Could you check a few things on this model? Use its own coordinates, in mm. A direction names the side the tool comes from. Coordinates: 2 decimals unless noted, no trailing zeros. Loops run counter-clockwise (first coordinate to the right, second up) from the corner with the lowest first, then second, coordinate; pieces in that order, holes last. Notation, with made-up numbers: (42.25, 40.25) - (101.25, 40.25) arc R30 cw to (101.25, 77.25) - close; hole circle Ø6 at (68.5, 56.5). An arc over 180 degrees is marked (long way). Use CSV: the item, a comma, the result in double quotes.
from build123d import *

# Parameters (mm, degrees)
BOSS_EXTRUDE1_DEPTH = 3
BOSS_EXTRUDE2_DEPTH = 13
FILLET1_R           = 10


with BuildPart() as part:
    # Sketch1 → Boss-Extrude1 (new body)
    with BuildSketch(Plane.XY):
        with BuildLine():
            ThreePointArc((44.504151191, -3.633742271), (52.754151191, 4.616257729), (61.004151191, -3.633742271))
            Line((61.004151191, -3.633742271), (71.117527312, -3.633742271))
            Line((71.117527312, -3.633742271), (71.117527312, 12.71809795))
            Line((71.117527312, 12.71809795), (-33.093009972, 12.71809795))
            Line((-33.093009972, 12.71809795), (-33.093009972, -3.633742271))
            Line((-33.093009972, -3.633742271), (-21.941421773, -3.633742271))
            ThreePointArc((-21.941421773, -3.633742271), (-13.691421773, 4.616257729), (-5.441421773, -3.633742271))
            Line((-5.441421773, -3.633742271), (10.76225867, -3.633742271))
            ThreePointArc((10.76225867, -3.633742271), (19.01225867, 4.616257729), (27.26225867, -3.633742271))
            Line((27.26225867, -3.633742271), (44.504151191, -3.633742271))
        make_face()
        with BuildLine():
            Line((71.117527312, -3.633742271), (61.004151191, -3.633742271))
            ThreePointArc((61.004151191, -3.633742271), (52.754151191, -11.883742271), (44.504151191, -3.633742271))
            Line((44.504151191, -3.633742271), (27.26225867, -3.633742271))
            ThreePointArc((27.26225867, -3.633742271), (19.01225867, -11.883742271), (10.76225867, -3.633742271))
            Line((10.76225867, -3.633742271), (-5.441421773, -3.633742271))
            ThreePointArc((-5.441421773, -3.633742271), (-13.691421773, -11.883742271), (-21.941421773, -3.633742271))
            Line((-21.941421773, -3.633742271), (-33.093009972, -3.633742271))
            Line((-33.093009972, -3.633742271), (-33.093009972, -19.985582493))
            Line((-33.093009972, -19.985582493), (71.117527312, -19.985582493))
            Line((71.117527312, -19.985582493), (71.117527312, -3.633742271))
        make_face()
        with BuildLine():
            ThreePointArc((-21.941421773, -3.633742271), (-13.691421773, -11.883742271), (-5.441421773, -3.633742271))
            Line((-5.441421773, -3.633742271), (-21.941421773, -3.633742271))
        make_face()
        with BuildLine():
            Line((-21.941421773, -3.633742271), (-5.441421773, -3.633742271))
            ThreePointArc((-5.441421773, -3.633742271), (-13.691421773, 4.616257729), (-21.941421773, -3.633742271))
        make_face()
        with BuildLine():
            ThreePointArc((10.76225867, -3.633742271), (19.01225867, -11.883742271), (27.26225867, -3.633742271))
            Line((27.26225867, -3.633742271), (10.76225867, -3.633742271))
        make_face()
        with BuildLine():
            Line((10.76225867, -3.633742271), (27.26225867, -3.633742271))
            ThreePointArc((27.26225867, -3.633742271), (19.01225867, 4.616257729), (10.76225867, -3.633742271))
        make_face()
        with BuildLine():
            ThreePointArc((44.504151191, -3.633742271), (52.754151191, -11.883742271), (61.004151191, -3.633742271))
            Line((61.004151191, -3.633742271), (44.504151191, -3.633742271))
        make_face()
        with BuildLine():
            Line((44.504151191, -3.633742271), (61.004151191, -3.633742271))
            ThreePointArc((61.004151191, -3.633742271), (52.754151191, 4.616257729), (44.504151191, -3.633742271))
        make_face()
    extrude(amount=BOSS_EXTRUDE1_DEPTH)

    # Sketch1_3 → Boss-Extrude2 (add)
    with BuildSketch(Plane.XY):
        with BuildLine():
            ThreePointArc((-21.941421773, -3.633742271), (-13.691421773, -11.883742271), (-5.441421773, -3.633742271))
            Line((-5.441421773, -3.633742271), (-21.941421773, -3.633742271))
        make_face()
        with BuildLine():
            Line((-21.941421773, -3.633742271), (-5.441421773, -3.633742271))
            ThreePointArc((-5.441421773, -3.633742271), (-13.691421773, 4.616257729), (-21.941421773, -3.633742271))
        make_face()
        with BuildLine():
            ThreePointArc((10.76225867, -3.633742271), (19.01225867, -11.883742271), (27.26225867, -3.633742271))
            Line((27.26225867, -3.633742271), (10.76225867, -3.633742271))
        make_face()
        with BuildLine():
            Line((10.76225867, -3.633742271), (27.26225867, -3.633742271))
            ThreePointArc((27.26225867, -3.633742271), (19.01225867, 4.616257729), (10.76225867, -3.633742271))
        make_face()
        with BuildLine():
            ThreePointArc((44.504151191, -3.633742271), (52.754151191, -11.883742271), (61.004151191, -3.633742271))
            Line((61.004151191, -3.633742271), (44.504151191, -3.633742271))
        make_face()
        with BuildLine():
            Line((44.504151191, -3.633742271), (61.004151191, -3.633742271))
            ThreePointArc((61.004151191, -3.633742271), (52.754151191, 4.616257729), (44.504151191, -3.633742271))
        make_face()
    extrude(amount=BOSS_EXTRUDE2_DEPTH)

    # Fillet1
    fillet1_edges = [part.edges().sort_by_distance(p)[0] for p in [
        (-33.093009972, -19.985582493, 1.5),
        (-33.093009972, 12.71809795, 1.5),
        (71.117527312, 12.71809795, 1.5),
        (71.117527312, -19.985582493, 1.5),
    ]]
    fillet(fillet1_edges, radius=FILLET1_R)

    # Fillet2: read off the stored shape, not the designer's step
    # Fillet2 outline → Fillet2 (revolve, cut)
    with BuildSketch(Plane(origin=(52.754151191, -3.633742271, 0), x_dir=(1, 0, 0), z_dir=(0, -1, 0))):
        with BuildLine():
            ThreePointArc((5.75, 13), (7.517766953, 12.267766953), (8.25, 10.5))
            Line((8.25, 10.5), (8.25, 13))
            Line((8.25, 13), (5.75, 13))
        make_face()
    revolve(axis=Axis((52.754151191, -3.633742271, 0), (0, 0, 1)), mode=Mode.SUBTRACT)

    # Fillet2 2 outline → Fillet2 2 (revolve, cut)
    with BuildSketch(Plane(origin=(19.01225867, -3.633742271, 0), x_dir=(1, 0, 0), z_dir=(0, -1, 0))):
        with BuildLine():
            ThreePointArc((5.75, 13), (7.517766953, 12.267766953), (8.25, 10.5))
            Line((8.25, 10.5), (8.25, 13))
            Line((8.25, 13), (5.75, 13))
        make_face()
    revolve(axis=Axis((19.01225867, -3.633742271, 0), (0, 0, 1)), mode=Mode.SUBTRACT)

    # Fillet2 3 outline → Fillet2 3 (revolve, cut)
    with BuildSketch(Plane(origin=(-13.691421773, -3.633742271, 0), x_dir=(1, 0, 0), z_dir=(0, -1, 0))):
        with BuildLine():
            ThreePointArc((5.75, 13), (7.517766953, 12.267766953), (8.25, 10.5))
            Line((8.25, 10.5), (8.25, 13))
            Line((8.25, 13), (5.75, 13))
        make_face()
    revolve(axis=Axis((-13.691421773, -3.633742271, 0), (0, 0, 1)), mode=Mode.SUBTRACT)


solid = part.part
(1) Suppose I cut it at B-B (z = 11.75). Write out the boundary of the cut face in (x, y).
Computed:
outline,"circle Ø15.83 at (-13.69, -3.63); circle Ø15.83 at (19.01, -3.63); circle Ø15.83 at (52.75, -3.63)"
(2) Thinking about a two-plate mould opening in X: for faces 3 (the face through (18, -19.986, 1)), 4 (the face through (-9.256, 3.323, 6.698)), 5 (the face through (71.118, -4, 1)), which applies, +X half, -X half, draft (parallel to the pull), parting line (faces both ways), or undercut?
Computed:
face 3,"draft"
face 4,"undercut"
face 5,"+X half"
(3) Please list where these lines run through material, in increasing order: line 1 (X direction, y = -9, z = 8.75); line 2 (X direction, y = -8.5, z = 6.5); line 3 (Z direction, x = 67.5, y = 0.5).
Computed:
line 1,"x = -19.96 to -7.43, 12.75 to 25.28, 46.49 to 59.02"
line 2,"x = -20.35 to -7.03, 12.35 to 25.67, 46.09 to 59.42"
line 3,"z = 0 to 3"
(4) Which directions (+Z, -Z, +X, -X, +Y, -Y) give clear straight access to the entire face, cutting with the end or side of a thin tool? Please do faces 1 (the face through (-30.086, 9.866, 1.521)), 2 (the face through (44.512, -3.271, 6.698)).
Computed:
face 1,"+Z, -Z, -X, +Y"
face 2,"+Z"
(5) Will these pins go through, and if not, where does the flat tip stop? pin 1 (10 mm diameter, centred on x = -4.5, y = -9.5, fed in from +Z); pin 2 (4 mm diameter, centred on x = 28.5, y = -13, fed in from +Z).
Computed:
pin 1,"stops at z = 13"
pin 2,"stops at z = 3"
(6) Suppose I cut it at C-C (y = -15.5). Write out the boundary of the cut face in (x, z).
Computed:
outline,"(-31.44, 0) - (69.46, 0) - (69.46, 3) - (-31.44, 3) - close"
(7) Suppose I cut it at A-A (x = 42). Write out the boundary of the cut face in (y, z), plus the area to 3 significant figures.
Computed:
outline,"(-19.99, 0) - (12.72, 0) - (12.72, 3) - (-19.99, 3) - close"
area,"98.1 mm²"
